Can you work these out from the model? Positions are in its coordinate system, mm. A direction names the side the tool comes from. Round coordinates to 2 decimals unless told otherwise and drop trailing zeros. Loops run counter-clockwise (first coordinate to the right, second up) from the corner with the lowest first, then second, coordinate; pieces in that order, holes last.
(1) If I drill on line 1 along Y through (x, z) = (-69.5, 17.5); line 2 along Z through (x, y) = (-87.5, -15); line 3 along X through (y, z) = (12.5, 12), over which ranges is the centre line in solid material (lowest first)?
(2) Will these pins go through, and if not, where does the flat tip stop? pin 1 Ø10 at (y, z) = (14.5, 0) entering from +X; pin 2 Ø4.5 at (y, z) = (18, -4) entering from +X; pin 3 Ø1.5 at (x, y) = (-20, 18) entering from -Z.
(3) I want a section at B-B on x = -49. Write out the boundary of the cut face in (y, z), plus the area to 3 significant figures.
(4) Which directions (+Z, -Z, +X, -X, +Y, -Y) give clear straight access to the entire face, cutting with the end or side of a thin tool? Please do faces 4 (the face through (-21.76, 14.4, 9.39)), 5 (the face through (-94.875, 13.586, -11.297)), 6 (the face through (-49, 4, 0)).
(5) I want a section at A-A on z = 12. Write out the boundary of the cut face in (x, y) (1 decimal).
(6) Thinking about a two-plate mould opening in X: for faces 1 (the face through (-75.732, 14.192, 9.392)), 2 (the face through (-1.93, 13.59, 3.29)), 3 (the face through (-51, 65.097, 7)), which applies, released by +X, released by -X, zero draft, split by the parting line, or undercut?
from build123d import *

# Parameters (mm, degrees)
F0_W     = 101.6
F0_H     = 101.6
F1_DEPTH = 19.05
F2_W     = 12.7
F2_H     = 101.6
F3_DEPTH = 11.43
F5_DEPTH = 101.601
F6_DEPTH = 101.601


with BuildPart() as f1:
    # F0 (on Top) → F1 (new body)
    with BuildSketch(Plane.XY):
        with Locations((-50.5425002087, 14.2971096218)):
            Rectangle(F0_W, F0_H)
        with BuildLine():
            ThreePointArc((-70.9710493684, 9.5346096218), (-75.7335493684, 14.2971096218), (-70.9710493684, 19.0596096218))
            Line((-70.9710493684, 19.0596096218), (-26.5210493684, 19.0596096218))
            ThreePointArc((-26.5210493684, 19.0596096218), (-21.7585493684, 14.2971096218), (-26.5210493684, 9.5346096218))
            Line((-26.5210493684, 9.5346096218), (-70.9710493684, 9.5346096218))
        make_face(mode=Mode.SUBTRACT)
    extrude(amount=F1_DEPTH)

    # F2 (on face) → F3 (join)
    with BuildSketch(Plane(origin=(0, 0, 0), x_dir=(1, 0, 0), z_dir=(0, 0, -1))):
        with Locations((-94.9925002087, -14.2971096218)):
            Rectangle(F2_W, F2_H)
    extrude(amount=F3_DEPTH)

    # F4 (on face) → F5 (cut, through all)
    with BuildSketch(Plane.XZ.offset(36.5028903782)):
        with BuildLine():
            ThreePointArc((0.2574997913, 9.2125750211), (-1.9847896018, 3.2247694582), (-7.5058890507, 0))
            Line((-7.5058890507, 0), (0.2574997913, 0))
            Line((0.2574997913, 0), (0.2574997913, 9.2125750211))
        make_face()
    extrude(amount=-F5_DEPTH, mode=Mode.SUBTRACT)

    # F4 (on face) → F6 (cut, through all)
    with BuildSketch(Plane.XZ.offset(36.5028903782)):
        with BuildLine():
            Line((-88.6425002087, -11.43), (-88.6425002087, -5.715))
            ThreePointArc((-88.6425002087, -5.715), (-95.0047463509, -11.2975338614), (-101.3425002087, -5.6872097775))
            Line((-101.3425002087, -5.6872097775), (-101.3425002087, -11.43))
            Line((-101.3425002087, -11.43), (-88.6425002087, -11.43))
        make_face()
    extrude(amount=-F6_DEPTH, mode=Mode.SUBTRACT)


solid = f1.part
Filled sheet:
1. line 1: y = -36.5 to 9.53, 19.06 to 65.1
1. line 2: z = 0 to 19.05
1. line 3: x = -101.34 to -75.38, -22.11 to 0.26
2. pin 1: stops at x = -0.8
2. pin 2: stops at x = -88.64
2. pin 3: stops at z = 0
3. outline: (-36.5, 0) - (9.53, 0) - (9.53, 19.05) - (-36.5, 19.05) - close; (19.06, 0) - (65.1, 0) - (65.1, 19.05) - (19.06, 19.05) - close
3. area: 1,750 mm2
4. face 4: +Z, -Z
4. face 5: -Z, +Y, -Y
4. face 6: -Z, +X, +Y, -Y
5. outline: (-101.3, -36.5) - (0.3, -36.5) - (0.3, 65.1) - (-101.3, 65.1) - close; hole (-71, 9.5) - (-26.5, 9.5) arc R4.8 ccw to (-26.5, 19.1) - (-71, 19.1) arc R4.8 ccw to start
6. face 1: undercut
6. face 2: released by +X
6. face 3: zero draft
